Input: part model. Units: mm. Frame: model coordinates. Face numbers are marked on the shaded views. A direction names the side the tool comes from. Coordinates: 2 decimals unless noted, no trailing zeros. Order: outer loops, then holes, each group sorted by start corner. A loop starts at its lowest first (then second) coordinate and runs counter-clockwise, first axis right, second up. Notation, with made-up numbers: M -6,37 L 39,37 A19 ccw 39,68 Z; hole C 2,28 d5. An arc over 180 degrees is marked long. One line per item, written item: value.
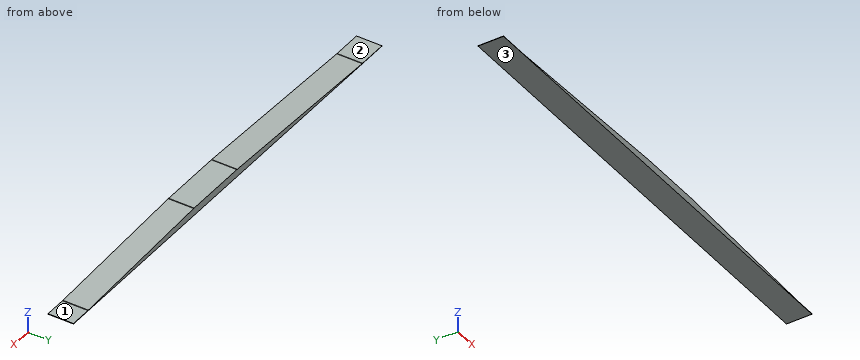
```python
from build123d import *

# Parameters (mm, degrees)
F1_DEPTH    = 107.95
F2_T1_DEPTH = 107.95
F3_T1_DEPTH = 107.95
F3_T3_DEPTH = 115.0912402897
F3_T5_DEPTH = 116.2011283703


# Not quite as in the source:
# - a fillet or chamfer that OpenCascade refuses, or shapes differently, is made with other operations: its cross-section is extruded or revolved along the edge and cut away or added


with BuildPart() as f1:
    # F0 (on Front) → F1 (new body)
    with BuildSketch(Plane.XZ):
        Polygon((-1016, 1.27), (-1016, 0), (984, 0), (984, 2.032), (889, 2.032), (203.2, 31.75), (-76.2, 31.75), (-889, 1.27), align=None)
    extrude(amount=F1_DEPTH)

    # F2: fillet of radius 76.2 on 1 edges, made by hand

    # F2_s2 → F2_t1 (join)
    with BuildSketch(Plane.XZ):
        with BuildLine():
            ThreePointArc((-887.5727551211, 1.323521683), (-889.0002508168, 1.2833815957), (-890.4282480579, 1.27))
            Line((-890.4282480579, 1.27), (-889, 1.27))
            Line((-889, 1.27), (-887.5727551211, 1.323521683))
        make_face()
    extrude(amount=F2_T1_DEPTH)

    # F3: fillet of radius 76.2 on 3 edges, made by hand

    # F3_s2 → F3_t1 (join)
    with BuildSketch(Plane.XZ):
        with BuildLine():
            ThreePointArc((890.6502256741, 2.032), (889.0003868453, 2.0498627772), (887.3513215259, 2.1034427339))
            Line((887.3513215259, 2.1034427339), (889, 2.032))
            Line((889, 2.032), (890.6502256741, 2.032))
        make_face()
    extrude(amount=F3_T1_DEPTH)

    # F3_s4 → F3_t3 (cut)
    with BuildSketch(Plane.XZ.offset(-3.5706201449)):
        with BuildLine():
            ThreePointArc((-77.6272448789, 31.696478317), (-76.1997491832, 31.7366184043), (-74.7717519421, 31.75))
            Line((-74.7717519421, 31.75), (-76.2, 31.75))
            Line((-76.2, 31.75), (-77.6272448789, 31.696478317))
        make_face()
    extrude(amount=F3_T3_DEPTH, mode=Mode.SUBTRACT)

    # F3_s6 → F3_t5 (cut)
    with BuildSketch(Plane.XZ.offset(-4.1255641851)):
        with BuildLine():
            ThreePointArc((201.5497743259, 31.75), (203.1996131547, 31.7321372228), (204.8486784741, 31.6785572661))
            Line((204.8486784741, 31.6785572661), (203.2, 31.75))
            Line((203.2, 31.75), (201.5497743259, 31.75))
        make_face()
    extrude(amount=F3_T5_DEPTH, mode=Mode.SUBTRACT)


solid = f1.part
```
(1) Access query for the marked faces 1, 2 and 3. Directions: +Z, -Z, +X, -X, +Y, -Y. A direction counts if a zero-diameter tool reaches every point of the face in a straight line with its end or side. Return the directions, or none.
Data:
face 1: +Z, +X, +Y, -Y
face 2: +Z, -X, +Y, -Y
face 3: -Z, +X, -X, +Y, -Y
(2) First-contact query: pin 1 (1 mm diameter, centred on x = 433.5, z = 23, fed in from +Y); pin 2 (1.5 mm diameter, centred on x = -381.5, y = -25, fed in from +Z). Flat tips, straight axial feed; report the tip coordinate or a pass-through.
Data:
pin 1: passes through
pin 2: stops at z = 20.33
(3) Ray query, line 1 (Z direction, x = 793, y = -29.5); line 2 (Z direction, x = -925, y = -27). Return the intervals inside material, ascending. Write a range as from..to.
Data:
line 1: z = 0..6.19
line 2: z = 0..1.27
(4) Cut plane A-A on y = -38. Output: boundary loops of the cut face in (x, z).
Data:
outline: M -1016,0 L 984,0 L 984,2.03 L 890.65,2.03 A76.2 cw 887.35,2.1 L 204.85,31.68 A76.2 ccw 201.55,31.75 L -74.77,31.75 A76.2 ccw -77.63,31.7 L -887.57,1.32 A76.2 cw -890.43,1.27 L -1016,1.27 Z
(5) Cut plane B-B on x = -385. Output: boundary loops of the cut face in (y, z).
Data:
outline: M -107.95,0 L 0,0 L 0,20.17 L -107.95,20.17 Z
(6) Cut plane C-C on z = 11.5. Output: boundary loops of the cut face in (x, y).
Data:
outline: M -616.2,-107.95 L 670.51,-107.95 L 670.51,0 L -616.2,0 Z
